The model under review builds one solid part; all positions refer to its coordinate system, in mm. A direction names the side the tool comes from. Round coordinates to 2 decimals unless told otherwise and drop trailing zeros.
1) Clearance check with flat-ended pins moving along their axes: P1, Ø1.2, axis at x = -5.77, y = 0, coming from the +Z side; P2, Ø3, axis at y = -37, z = 6, coming from the +X side; P3, Ø2, axis at x = 15, y = -19.5, coming from the -Z side. State where each tip first meets the part, or that it passes through.
2) To check wall thickness, follow L1, parallel to Y at x = 20, z = 5; L2, parallel to Y at x = -54.5, z = 3.25; L3, parallel to X at y = -44, z = 0.5. State the ranges of each line that lie inside material, in increasing order.
3) Mouldability with a two-part tool opening along Y and no side actions: class faces 1 (the face through (-31, 42, 0)), 2 (the face through (-0.759, -17.417, 2.218)), 3 (the face through (-47.7, 27.1, 0.6)), 4 (the face through (47.7, -27.04, 6.43)) as pulls with the +Y half, pulls with the -Y half, needs draft (parallel to the pull), parting line crosses it, or undercut.
4) Machinability: for faces 5 (the face through (-51, 6, 0)), 6 (the face through (-18.263, -51.535, 2.218)), which of the approach directions +Z, -Z, +X, -X, +Y, -Y give a long, thin tool a straight path to every point of the face, cutting with its end or side? Answer none if there is none.
from build123d import *

# Parameters (mm, degrees)
F0_R     = 1
F1_DEPTH = 7
F2_T     = -2.5
F3_R     = 2
F5_DEPTH = 25
F6_DEPTH = 25


with BuildPart() as f1:
    # F0 (on Top) → F1 (new body)
    with BuildSketch(Plane.XY):
        Polygon((0, 0), (-32.0025254212, 55.43), (-64.0050508424, 0), (-32.0025254212, -55.43), (32.0025254212, -55.43), (64.0050508424, 0), (32.0025254212, 55.43), align=None)
        with Locations((-32.0025254212, -41.43)):
            Circle(F0_R, mode=Mode.SUBTRACT)
        with Locations((-19.8781697682, -48.43)):
            Circle(F0_R, mode=Mode.SUBTRACT)
        with Locations((-51.8806951894, -7)):
            Circle(F0_R, mode=Mode.SUBTRACT)
        with Locations((-12.124355653, -7)):
            Circle(F0_R, mode=Mode.SUBTRACT)
        with Locations((19.8781697682, -48.43)):
            Circle(F0_R, mode=Mode.SUBTRACT)
        with Locations((32.0025254212, -41.43)):
            Circle(F0_R, mode=Mode.SUBTRACT)
        with Locations((0, -14)):
            Circle(F0_R, mode=Mode.SUBTRACT)
        with Locations((12.124355653, -7)):
            Circle(F0_R, mode=Mode.SUBTRACT)
        with Locations((51.8806951894, -7)):
            Circle(F0_R, mode=Mode.SUBTRACT)
        with Locations((-51.8806951894, 7)):
            Circle(F0_R, mode=Mode.SUBTRACT)
        with Locations((-12.124355653, 7)):
            Circle(F0_R, mode=Mode.SUBTRACT)
        with Locations((-32.0025254212, 41.43)):
            Circle(F0_R, mode=Mode.SUBTRACT)
        with Locations((12.124355653, 7)):
            Circle(F0_R, mode=Mode.SUBTRACT)
        with Locations((51.8806951894, 7)):
            Circle(F0_R, mode=Mode.SUBTRACT)
        with Locations((32.0025254212, 41.43)):
            Circle(F0_R, mode=Mode.SUBTRACT)
        with BuildLine():
            Line((0, 55.43), (-32.0025254212, 55.43))
            Line((-32.0025254212, 55.43), (0, 0))
            Line((0, 0), (0, 13))
            ThreePointArc((0, 13), (-0.9659258263, 13.7411809549), (-0.5, 14.8660254038))
            Line((-0.5, 14.8660254038), (-19.3781697682, 47.5639745962))
            ThreePointArc((-19.3781697682, 47.5639745962), (-20.744195172, 48.93), (-18.8781697682, 48.43))
            Line((-18.8781697682, 48.43), (0, 48.43))
            Line((0, 48.43), (0, 55.43))
        make_face()
        with BuildLine():
            Line((32.0025254212, 55.43), (0, 55.43))
            Line((0, 55.43), (0, 48.43))
            Line((0, 48.43), (18.8781697682, 48.43))
            ThreePointArc((18.8781697682, 48.43), (19.8781697682, 49.43), (20.8781697682, 48.43))
            ThreePointArc((20.8781697682, 48.43), (20.3781697682, 47.5639745962), (19.3781697682, 47.5639745962))
            Line((19.3781697682, 47.5639745962), (0.5, 14.8660254038))
            ThreePointArc((0.5, 14.8660254038), (0.8660254038, 14.5), (1, 14))
            ThreePointArc((1, 14), (0.7071067812, 13.2928932188), (0, 13))
            Line((0, 13), (0, 0))
            Line((0, 0), (32.0025254212, 55.43))
        make_face()
        with BuildLine():
            Line((0, 15), (0, 48.43))
            Line((0, 48.43), (-18.8781697682, 48.43))
            ThreePointArc((-18.8781697682, 48.43), (-19.0121443644, 47.93), (-19.3781697682, 47.5639745962))
            Line((-19.3781697682, 47.5639745962), (-0.5, 14.8660254038))
            ThreePointArc((-0.5, 14.8660254038), (-0.2588190451, 14.9659258263), (0, 15))
        make_face()
        with BuildLine():
            Line((18.8781697682, 48.43), (0, 48.43))
            Line((0, 48.43), (0, 15))
            ThreePointArc((0, 15), (0.2588190451, 14.9659258263), (0.5, 14.8660254038))
            Line((0.5, 14.8660254038), (19.3781697682, 47.5639745962))
            ThreePointArc((19.3781697682, 47.5639745962), (19.0121443644, 47.93), (18.8781697682, 48.43))
        make_face()
    extrude(amount=F1_DEPTH)

    # F2
    f2_openings = [f1.faces().sort_by_distance(p)[0] for p in [
        (0, 0, 0),
    ]]
    offset(amount=F2_T, openings=f2_openings)

    # F3
    f3_edges = [f1.edges().sort_by_distance(p)[0] for p in [
        (0, -55.43, 7),
        (-48.003788, -27.715, 7),
        (-48.003788, 27.715, 7),
        (0, 55.43, 7),
        (48.003788, 27.715, 7),
        (48.003788, -27.715, 7),
        (48.003788, -27.715, 0),
        (0, -55.43, 0),
        (32.002525, -55.43, 3.5),
        (64.005051, 0, 3.5),
        (48.003788, 27.715, 0),
        (32.002525, 55.43, 3.5),
        (0, 55.43, 0),
        (-32.002525, 55.43, 3.5),
        (-48.003788, 27.715, 0),
        (-64.005051, 0, 3.5),
        (-48.003788, -27.715, 0),
        (-32.002525, -55.43, 3.5),
    ]]
    fillet(f3_edges, radius=F3_R)

    # F4 (on face) → F5 (cut)
    with BuildSketch(Plane.XY.offset(7)):
        with BuildLine():
            Line((-1.8867513459, 5), (-2.8867513459, 5))
            Line((-2.8867513459, 5), (-3.3867513459, 4.1339745962))
            ThreePointArc((-3.3867513459, 4.1339745962), (-2.3867513459, 4.1339745962), (-1.8867513459, 5))
        make_face()
        with BuildLine():
            Line((-3.3867513459, 4.1339745962), (-2.8867513459, 5))
            Line((-2.8867513459, 5), (-1.8867513459, 5))
            ThreePointArc((-1.8867513459, 5), (-3.3867513459, 5.8660254038), (-3.3867513459, 4.1339745962))
        make_face()
    extrude(amount=-F5_DEPTH, mode=Mode.SUBTRACT)

    # F4 (on face) → F6 (cut)
    with BuildSketch(Plane.XY.offset(7)):
        with BuildLine():
            Line((-3.3867513459, 4.1339745962), (-2.8867513459, 5))
            Line((-2.8867513459, 5), (-1.8867513459, 5))
            ThreePointArc((-1.8867513459, 5), (-3.3867513459, 5.8660254038), (-3.3867513459, 4.1339745962))
        make_face()
        with BuildLine():
            Line((-1.8867513459, 5), (-2.8867513459, 5))
            Line((-2.8867513459, 5), (-3.3867513459, 4.1339745962))
            ThreePointArc((-3.3867513459, 4.1339745962), (-2.3867513459, 4.1339745962), (-1.8867513459, 5))
        make_face()
        with BuildLine():
            Line((-5.7735026919, 0), (-5.2735026919, 0.8660254038))
            ThreePointArc((-5.2735026919, 0.8660254038), (-6.7735026919, 0), (-5.2735026919, -0.8660254038))
            Line((-5.2735026919, -0.8660254038), (-5.7735026919, 0))
        make_face()
        with BuildLine():
            ThreePointArc((-4.7735026919, 0), (-4.9074772881, 0.5), (-5.2735026919, 0.8660254038))
            Line((-5.2735026919, 0.8660254038), (-5.7735026919, 0))
            Line((-5.7735026919, 0), (-5.2735026919, -0.8660254038))
            ThreePointArc((-5.2735026919, -0.8660254038), (-4.9074772881, -0.5), (-4.7735026919, 0))
        make_face()
        with BuildLine():
            Line((-2.8867513459, -5), (-3.3867513459, -4.1339745962))
            ThreePointArc((-3.3867513459, -4.1339745962), (-3.3867513459, -5.8660254038), (-1.8867513459, -5))
            Line((-1.8867513459, -5), (-2.8867513459, -5))
        make_face()
        with BuildLine():
            ThreePointArc((-1.8867513459, -5), (-2.3867513459, -4.1339745962), (-3.3867513459, -4.1339745962))
            Line((-3.3867513459, -4.1339745962), (-2.8867513459, -5))
            Line((-2.8867513459, -5), (-1.8867513459, -5))
        make_face()
        with BuildLine():
            ThreePointArc((3.8867513459, -5), (3.7527767497, -4.5), (3.3867513459, -4.1339745962))
            Line((3.3867513459, -4.1339745962), (2.8867513459, -5))
            Line((2.8867513459, -5), (1.8867513459, -5))
            ThreePointArc((1.8867513459, -5), (2.8867513459, -6), (3.8867513459, -5))
        make_face()
        with BuildLine():
            Line((2.8867513459, -5), (3.3867513459, -4.1339745962))
            ThreePointArc((3.3867513459, -4.1339745962), (2.3867513459, -4.1339745962), (1.8867513459, -5))
            Line((1.8867513459, -5), (2.8867513459, -5))
        make_face()
        with BuildLine():
            ThreePointArc((6.7735026919, 0), (6.2735026919, 0.8660254038), (5.2735026919, 0.8660254038))
            Line((5.2735026919, 0.8660254038), (5.7735026919, 0))
            Line((5.7735026919, 0), (5.2735026919, -0.8660254038))
            ThreePointArc((5.2735026919, -0.8660254038), (6.2735026919, -0.8660254038), (6.7735026919, 0))
        make_face()
        with BuildLine():
            Line((5.7735026919, 0), (5.2735026919, 0.8660254038))
            ThreePointArc((5.2735026919, 0.8660254038), (4.7735026919, 0), (5.2735026919, -0.8660254038))
            Line((5.2735026919, -0.8660254038), (5.7735026919, 0))
        make_face()
        with BuildLine():
            Line((2.8867513459, 5), (1.8867513459, 5))
            ThreePointArc((1.8867513459, 5), (2.3867513459, 4.1339745962), (3.3867513459, 4.1339745962))
            Line((3.3867513459, 4.1339745962), (2.8867513459, 5))
        make_face()
        with BuildLine():
            ThreePointArc((3.8867513459, 5), (2.8867513459, 6), (1.8867513459, 5))
            Line((1.8867513459, 5), (2.8867513459, 5))
            Line((2.8867513459, 5), (3.3867513459, 4.1339745962))
            ThreePointArc((3.3867513459, 4.1339745962), (3.7527767497, 4.5), (3.8867513459, 5))
        make_face()
    extrude(amount=-F6_DEPTH, mode=Mode.SUBTRACT)


solid = f1.part
Answer below:
1. P1: passes through
1. P2: stops at x = 43.39
1. P3: stops at z = 4.5
2. L1: y = -55.43 to -49.42, -47.44 to 47.44, 49.42 to 55.43
2. L2: y = -16.46 to -11.46, -9.32 to -4.68, 4.68 to 9.32, 11.46 to 16.46
2. L3: x = -37.82 to -35.71, -34.38 to -29.63, 29.63 to 34.38, 35.71 to 37.82
3. face 1: needs draft
3. face 2: undercut
3. face 3: pulls with the +Y half
3. face 4: pulls with the -Y half
4. face 5: -Z, +X, -X, +Y, -Y
4. face 6: -Z
